Source: three-view drawing plus pictorial views. Frame: mm from the lowest corner of the part. Coordinates: 2 decimals unless noted, no trailing zeros. Order: outer loops, then holes, each group sorted by start corner. A loop starts at its lowest first (then second) coordinate and runs counter-clockwise, first axis right, second up. Notation, with made-up numbers: (-22, -30) - (23, -30) arc R15 cw to (23, -10) - close; hole circle Ø5 at (51, 25). An arc over 180 degrees is marked (long way). One line per question, with ' | ' between items.
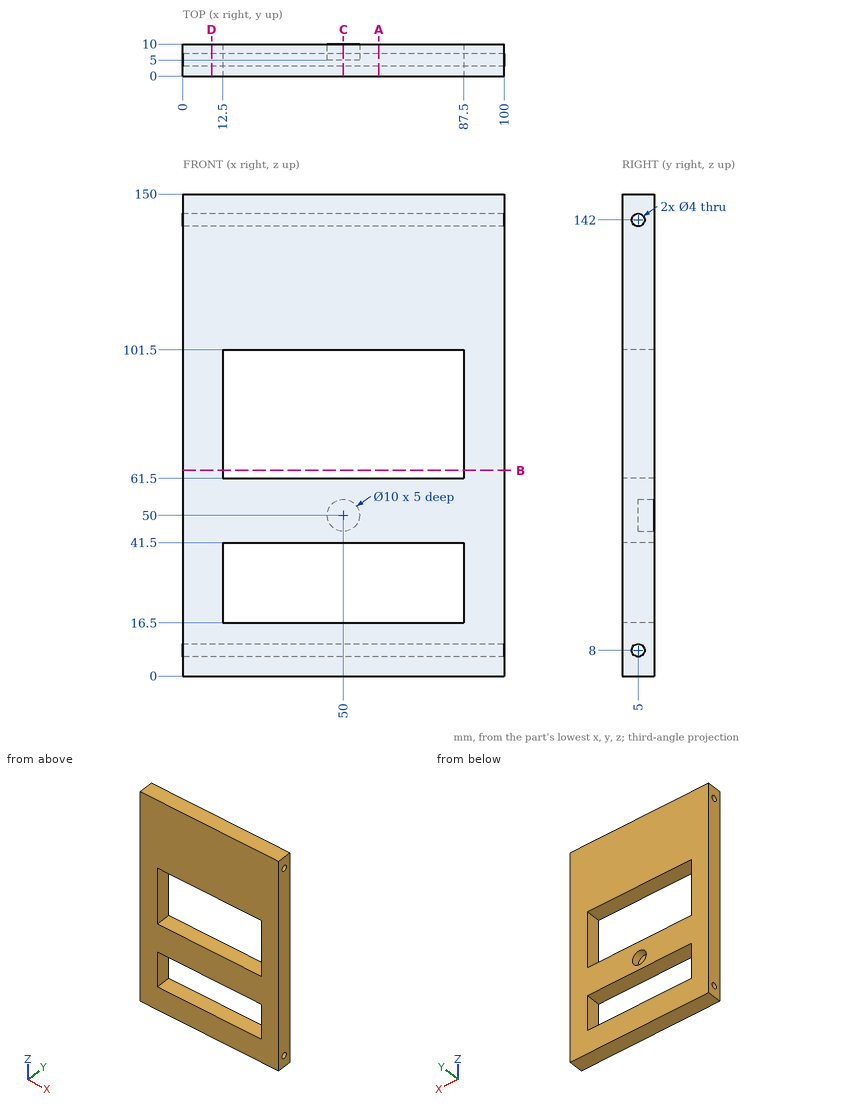
(1) Pin query (flat end, axial travel): P1, Ø6, axis at x = 50, z = 50, coming from the +Y side; P2, Ø3.5, axis at y = 5, z = 142, coming from the -X side. Return the tip coordinate at first contact, or that it passes through.
Taken from the geometry:
P1: stops at y = 5 | P2: passes through
(2) Cut plane C-C (x = 50). Return the cut outline in (y, z).
Taken from the geometry:
outline: (0, 0) - (10, 0) - (10, 16.5) - (0, 16.5) - close; (0, 41.5) - (10, 41.5) - (10, 45) - (5, 45) - (5, 55) - (10, 55) - (10, 61.5) - (0, 61.5) - close; (0, 101.5) - (10, 101.5) - (10, 150) - (0, 150) - close; hole circle Ø4 at (5, 8); hole circle Ø4 at (5, 142)
(3) Cut plane A-A (x = 61). Return the cut outline in (y, z).
Taken from the geometry:
outline: (0, 0) - (10, 0) - (10, 16.5) - (0, 16.5) - close; (0, 41.5) - (10, 41.5) - (10, 61.5) - (0, 61.5) - close; (0, 101.5) - (10, 101.5) - (10, 150) - (0, 150) - close; hole circle Ø4 at (5, 8); hole circle Ø4 at (5, 142)
(4) Material intervals for L1, parallel to Z at x = 80, y = 9; L2, parallel to Z at x = 50, y = 8.5; L3, parallel to X at y = 6, z = 50, sorted ascending. Write a range as from..to.
Taken from the geometry:
L1: z = 0..16.5, 41.5..61.5, 101.5..150 | L2: z = 0..16.5, 41.5..45, 55..61.5, 101.5..150 | L3: x = 0..45, 55..100
(5) Cut plane B-B (z = 64). Return the cut outline in (x, y).
Taken from the geometry:
outline: (0, 0) - (12.5, 0) - (12.5, 10) - (0, 10) - close; (87.5, 0) - (100, 0) - (100, 10) - (87.5, 10) - close
(6) Cut plane D-D (x = 9). Return the cut outline in (y, z), and give its area (3 significant figures).
Taken from the geometry:
outline: (0, 0) - (10, 0) - (10, 150) - (0, 150) - close; hole circle Ø4 at (5, 8); hole circle Ø4 at (5, 142) | area: 1,470 mm²
